Here's how the part is built. I have some questions about the finished solid (model axes, mm). Face numbers are marked on the shaded views. Coordinates: 2 decimals unless noted, no trailing zeros. Write each loop counter-clockwise with the first axis right and the second up, starting at its lowest first coordinate (ties: lowest second). Pieces come first, ordered by that corner, then holes.
Item 1: Please list where these lines run through material, in increasing order: line 1 (Y direction, x = 1.95, z = 0); line 2 (Y direction, x = 0.75, z = 0.5); line 3 (Y direction, x = 1.8, z = 3).
Item 2: I want a section at A-A (x = 0.6). Please give me the cut outline in (y, z).
Item 3: I'm going to push a flat-ended pin straight in: P1, Ø2, axis at y = 1, z = 1, coming from the -X side. Where does the tip first touch, or does it pass through?
Item 4: If we mould it in two halves opening along Y, with no side actions, what happens to the marked faces 1, 2, 3 and 4? For each: pulls with the +Y half, pulls with the -Y half, needs draft (parallel to the pull), parting line crosses it, or undercut.
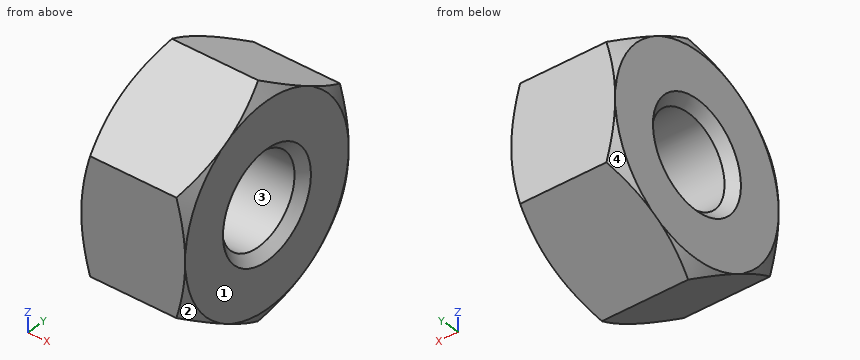
Autodesk Inventor part; units mm, degrees
ref_plane "MSC_PT1" through (2.9, 0, 0) normal (1, 0, 0) x (0, 1, 0)
ref_plane "MSC_PT2" through (0, 0, 0) normal (-1, 0, 0) x (0, -1, 0)
ref_plane "MSC_PF1" through (0, 0, 0) normal (1, 0, 0) x (0, 1, 0)
sketch "Boceto1" plane through (0, 0, 0) normal (1, 0, 0) x (0, 1, 0)
  line L0 (2.75, 1.5877) -> (2.75, -1.5877)
  line L1 (2.75, -1.5877) -> (0, -3.1754)
  line L2 (0, -3.1754) -> (-2.75, -1.5877)
  line L3 (-2.75, -1.5877) -> (-2.75, 1.5877)
  line L4 (-2.75, 1.5877) -> (0, 3.1754)
  line L5 (0, 3.1754) -> (2.75, 1.5877)
  circle A0 centre (0, 0) radius 2.75 construction
  dimension "d0" = 5.5
extrude "Extrusión1" add sketch "Boceto1" along normal blind 2.9
sketch "Boceto2" plane through (2.9, 0, 0) normal (1, 0, 0) x (0, 1, 0)
  line L0 (-2.75, 1.5877) -> (0, 3.1754)
  line L1 (0, -3.1754) -> (-2.75, -1.5877)
  line L2 (-2.75, 1.5877) -> (2.75, -1.5877) construction
  line L3 (-2.75, -1.5877) -> (2.75, 1.5877) construction
  point P0 (0, 0)
hole "Agujero1" at (2.9, 0, 0) direction (-1, 0, 0) diameter 2.459 end through all
chamfer "Chaflán1" distance 0.25 angle 45 2 edges at (2.9, 0, 1.2295) (0, 0, 1.2295)
sketch "Boceto3" plane through (0, 0, 0) normal (0, 1, 0) x (-1, 0, 0)
  line L0 (-7.0172, 0) -> (2.1698, 0)
  line L1 (-5.7048, 0) -> (0.8574, 0)
  line L2 (-2.9, 0) -> (-2.9, -3.1754)
  line L3 (-2.9, -3.1754) -> (0, -3.1754)
  line L4 (0, -3.1754) -> (0, 0)
  line L5 (-2.9, -1.5877) -> (-2.9, -3.1754)
  line L6 (0, -1.5877) -> (0, -3.1754)
  line L7 (0, -3.1754) -> (-2.9, -3.1754)
  line L8 (-2.9, -2.75) -> (-2.6544, -3.1754)
  line L9 (-2.9, -3.1754) -> (-2.9, -2.75)
  line L10 (-2.9, -3.1754) -> (-2.6544, -3.1754)
  line L11 (0, -2.75) -> (-0.2456, -3.1754)
  line L12 (-0.2456, -3.1754) -> (0, -3.1754)
  line L13 (0, -3.1754) -> (0, -2.75)
  dimension "d32" = 2.75
  dimension "d33" = 30
revolve "Revolución1" cut sketch "Boceto3" angle 360 about axis through (0, 0, 0) along (-1, 0, 0) contours L8 L3 L2 | L4 L3 L11
ref_plane "MSC_PT1" through (2.9, 0, 0) normal (1, 0, 0) x (0, 1, 0)
ref_plane "MSC_PT2" through (0, 0, 0) normal (-1, 0, 0) x (0, -1, 0)
ref_plane "MSC_PF1" through (0, 0, 0) normal (1, 0, 0) x (0, 1, 0)
equation "\"d0\" = Smax"
equation "\"d1\" = Mmax"
equation "\"d10\" = 0.5 * PTC"
equation "\"d32\" = 0.5 * Smax"
equation "\"NND\" = 3"
equation "\"Smax\" = 5.5"
equation "\"Mmax\" = 2.9"
equation "\"PTC\" = 0.5"
equation "\"THREADDIA\" = NND"
equation "\"TEMPLATE\" = 1.2345"
properties part number "ANSI B18.2.4.2M - M3x0,5" material "Acero, suave"
Answer:
1. line 1: y = -2.75 to -1.23, 1.23 to 2.75
1. line 2: y = -2.75 to -1.12, 1.12 to 2.75
1. line 3: y = -0.3 to 0.3
2. outline: (-2.75, -1.59) - (0, -3.18) - (2.75, -1.59) - (2.75, 1.59) - (0, 3.18) - (-2.75, 1.59) - close; hole circle Ø2.46 at (0, 0)
3. P1: stops at x = 0
4. face 1: needs draft
4. face 2: pulls with the -Y half
4. face 3: undercut
4. face 4: pulls with the +Y half
